```python
from build123d import *

# Parameters (mm, degrees)
F0_R     = 1.4224
F1_DEPTH = 12.7
F2_R     = 2.7051
F3_DEPTH = 1.4986
F4_R     = 1.27
F6_DEPTH = 0.89154


with BuildPart() as f1:
    # F0 (on Top) → F1 (new body)
    with BuildSketch(Plane.XY):
        Circle(F0_R)
    extrude(amount=F1_DEPTH)

    # F2 (on face) → F3 (join)
    with BuildSketch(Plane.XY.offset(12.7)):
        Circle(F2_R)
    extrude(amount=F3_DEPTH)

    # F4
    f4_edges = [f1.edges().sort_by_distance(p)[0] for p in [
        (-2.7051, 0, 14.1986),
    ]]
    fillet(f4_edges, radius=F4_R)

    # F5 (on face) → F6 (cut)
    with BuildSketch(Plane.XY.offset(14.1986)):
        Polygon((0.458272, -0.79375), (0.916544, 0), (0.458272, 0.79375), (-0.458272, 0.79375), (-0.916544, 0), (-0.458272, -0.79375), align=None)
    extrude(amount=-F6_DEPTH, mode=Mode.SUBTRACT)


solid = f1.part
```
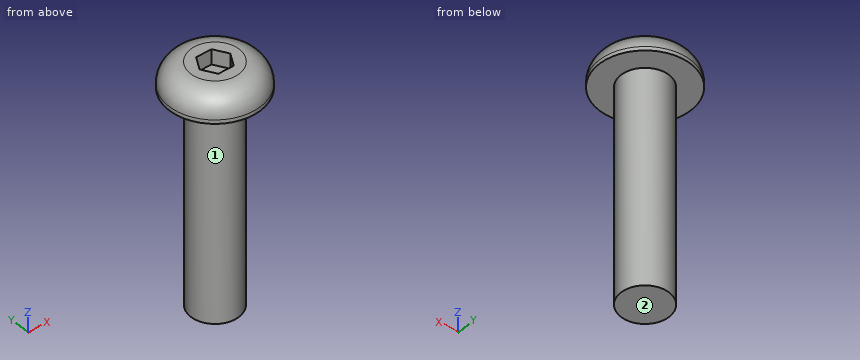
Input: part model. Units: mm. Frame: model coordinates. Face numbers are marked on the shaded views. A direction names the side the tool comes from. Give positions to 0.01 mm unless a question says otherwise; leave off trailing zeros. Order: outer loops, then holes, each group sorted by start corner. A loop starts at its lowest first (then second) coordinate and runs counter-clockwise, first axis right, second up. Notation, with made-up numbers: M 53.25,86 L 66.25,86 A28 cw 66.25,107 Z; hole C -11,37 d1. An arc over 180 degrees is marked long. Return JSON: item names as keys, results as strings.
1) Section query B-B on z = 1.25. Output: boundary loops of the cut face in (x, y), and give its area (3 significant figures).
Taken from the geometry:
{"outline": "C 0,0 d2.84", "area": "6.36 mm2"}
2) Line query: L1, parallel to Z at x = 1, y = -1.05; L2, parallel to Y at x = -0.1, z = 11.75; L3, parallel to Y at x = 1.25, z = 5.75. Output: solid intervals per line, ascending. Write a range as [from, to].
Taken from the geometry:
{"L1": "z = [12.7, 14.2]", "L2": "y = [-1.42, 1.42]", "L3": "y = [-0.68, 0.68]"}
3) Section query A-A on x = 0. Output: boundary loops of the cut face in (y, z), and give its area (3 significant figures).
Taken from the geometry:
{"outline": "M -2.71,12.7 L -1.42,12.7 L -1.42,0 L 1.42,0 L 1.42,12.7 L 2.71,12.7 L 2.71,12.93 A1.27 ccw 1.44,14.2 L 0.79,14.2 L 0.79,13.31 L -0.79,13.31 L -0.79,14.2 L -1.44,14.2 A1.27 ccw -2.71,12.93 Z", "area": "42.1 mm2"}
4) Contact query for flat-ended pins moving along their axis: pin 1 (1 mm diameter, centred on x = 0, z = 14, fed in from +Y); pin 2 (1.5 mm diameter, centred on x = 1.5, y = 0.5, fed in from +Z); pin 3 (1.5 mm diameter, centred on y = -1, z = 11.5, fed in from +X); pin 4 (1 mm diameter, centred on y = 1, z = 2, fed in from -X). Output: stop coordinate, or through.
Taken from the geometry:
{"pin 1": "stops at y = 2.57", "pin 2": "stops at z = 14.2", "pin 3": "stops at x = 1.4", "pin 4": "stops at x = -1.33"}
5) Access query for the marked faces 1 and 2. Directions: +Z, -Z, +X, -X, +Y, -Y. A direction counts if a zero-diameter tool reaches every point of the face in a straight line with its end or side. Return the directions, or none.
Taken from the geometry:
{"face 1": "-Z", "face 2": "-Z, +X, -X, +Y, -Y"}
